```python
from build123d import *

# Parameters (mm, degrees)
F0_R      = 3
F0_R_2    = 13
F1_DEPTH  = 2
F2_R      = 14
F2_R_2    = 12.75
F3_DEPTH  = 2.5
F4_R      = 14
F5_DEPTH  = 2
F7_DEPTH  = 2.5
F9_DEPTH  = 2
F11_DEPTH = 4.5
F12_R     = 24.5
F13_DEPTH = 1


with BuildPart() as f1:
    # F0 (on Top) → F1 (new body)
    with BuildSketch(Plane.XY):
        with BuildLine():
            ThreePointArc((-15, 21.236761), (-26, 0), (-15, -21.236761))
            ThreePointArc((-15, -21.236761), (0, -26), (15, -21.236761))
            ThreePointArc((15, -21.236761), (26, 0), (15, 21.236761))
            ThreePointArc((15, 21.236761), (0, 26), (-15, 21.236761))
        make_face()
        with Locations((0, -19)):
            Circle(F0_R, mode=Mode.SUBTRACT)
        Circle(F0_R_2, mode=Mode.SUBTRACT)
        with Locations((0, 19)):
            Circle(F0_R, mode=Mode.SUBTRACT)
    extrude(amount=F1_DEPTH)

    # F2 (on face) → F3 (join)
    with BuildSketch(Plane.XY.offset(2)):
        Circle(F2_R)
        Circle(F2_R_2, mode=Mode.SUBTRACT)
    extrude(amount=F3_DEPTH)

    # F4 (on face) → F5 (join)
    with BuildSketch(Plane.XY.offset(4.5)):
        Circle(F4_R)
    extrude(amount=F5_DEPTH)

    # F6 (on face) → F7 (join)
    with BuildSketch(Plane.XY.offset(2)):
        with BuildLine():
            Line((23.558438, -11), (19.627786, -11))
            ThreePointArc((19.627786, -11), (22.365353, 2.457846), (16.77051, 15))
            Line((16.77051, 15), (13.228757, 15))
            ThreePointArc((13.228757, 15), (20, 0), (13.228757, -15))
            Line((13.228757, -15), (16.77051, -15))
            Line((16.77051, -15), (21.236761, -15))
            ThreePointArc((21.236761, -15), (22.486717, -13.051726), (23.558438, -11))
        make_face()
        with BuildLine():
            Line((-13.228757, 15), (-16.77051, 15))
            Line((-16.77051, 15), (-21.236761, 15))
            ThreePointArc((-21.236761, 15), (-22.486717, 13.051726), (-23.558438, 11))
            Line((-23.558438, 11), (-19.627786, 11))
            ThreePointArc((-19.627786, 11), (-22.365353, -2.457846), (-16.77051, -15))
            Line((-16.77051, -15), (-13.228757, -15))
            ThreePointArc((-13.228757, -15), (-20, 0), (-13.228757, 15))
        make_face()
    extrude(amount=F7_DEPTH)

    # F8 (on face) → F9 (join)
    with BuildSketch(Plane.XY.offset(4.5)):
        with BuildLine():
            Line((-13.228757, 15), (-21.236761, 15))
            ThreePointArc((-21.236761, 15), (-26, 0), (-21.236761, -15))
            Line((-21.236761, -15), (-13.228757, -15))
            ThreePointArc((-13.228757, -15), (-20, 0), (-13.228757, 15))
        make_face()
        with BuildLine():
            ThreePointArc((21.236761, -15), (26, 0), (21.236761, 15))
            Line((21.236761, 15), (13.228757, 15))
            ThreePointArc((13.228757, 15), (20, 0), (13.228757, -15))
            Line((13.228757, -15), (21.236761, -15))
        make_face()
    extrude(amount=F9_DEPTH)

    # F10 (on face) → F11 (join)
    with BuildSketch(Plane.XY.offset(2)):
        with BuildLine():
            ThreePointArc((-9.177223, 13.106433), (-7.387978, 14.192173), (-5.472322, 15.035082))
            Line((-5.472322, 15.035082), (-7.695453, 21.143084))
            ThreePointArc((-7.695453, 21.143084), (-10.389344, 19.957744), (-12.90547, 18.430921))
            Line((-12.90547, 18.430921), (-9.177223, 13.106433))
        make_face()
        with BuildLine():
            Line((7.695453, 21.143084), (5.472322, 15.035082))
            ThreePointArc((5.472322, 15.035082), (7.387978, 14.192173), (9.177223, 13.106433))
            Line((9.177223, 13.106433), (12.90547, 18.430921))
            ThreePointArc((12.90547, 18.430921), (10.389344, 19.957744), (7.695453, 21.143084))
        make_face()
        with BuildLine():
            Line((-7.695453, -21.143084), (-5.472322, -15.035082))
            ThreePointArc((-5.472322, -15.035082), (-7.387978, -14.192173), (-9.177223, -13.106433))
            Line((-9.177223, -13.106433), (-12.90547, -18.430921))
            ThreePointArc((-12.90547, -18.430921), (-10.389344, -19.957744), (-7.695453, -21.143084))
        make_face()
        with BuildLine():
            ThreePointArc((9.177223, -13.106433), (7.387978, -14.192173), (5.472322, -15.035082))
            Line((5.472322, -15.035082), (7.695453, -21.143084))
            ThreePointArc((7.695453, -21.143084), (10.389344, -19.957744), (12.90547, -18.430921))
            Line((12.90547, -18.430921), (9.177223, -13.106433))
        make_face()
    extrude(amount=F11_DEPTH)

    # F12 (on face) → F13 (cut)
    with BuildSketch(Plane.XY.offset(6.5)):
        Circle(F12_R)
    extrude(amount=-F13_DEPTH, mode=Mode.SUBTRACT)


solid = f1.part
```
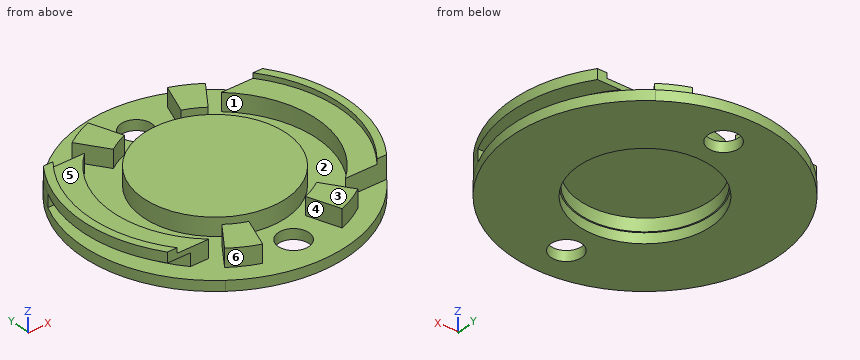
The model under review builds one solid part; all positions refer to its coordinate system, in mm. Face numbers are marked on the shaded views. A direction names the side the tool comes from. Round coordinates to 2 decimals unless told otherwise and drop trailing zeros. Loops run counter-clockwise (first coordinate to the right, second up) from the corner with the lowest first, then second, coordinate; pieces in that order, holes last. Notation, with made-up numbers: (19.25, 3.5) -> (23.25, 3.5) arc R20 ccw to (23.25, 8.5) -> close; hole circle Ø6 at (-21, 14). An arc over 180 degrees is marked (long way). Answer as a JSON object with one key per item and string values. Group by question number.
1) Mouldability with a two-part tool opening along Z and no side actions: class the marked faces 1, 2 and 3 as released by +Z, released by -Z, zero draft, split by the parting line, or undercut.
2) For line 1 (Y direction, x = 0, z = 0.6); line 2 (X direction, y = -0.5, z = 3); line 3 (Y direction, x = -11, z = 2.75), list the stretches that pass through material, from the lowest coordinate up. Write a range as [from, to].
3) For pin 1 Ø2 at (x, y) = (8, 16.5) entering from +Z; pin 2 Ø1 at (x, z) = (-5, 1) entering from +Y; pin 3 Ø13 at (x, y) = (2, 0) entering from -Z; pin 4 Ø10 at (x, y) = (-23, 0) entering from -Z, all flat-tipped, find the tip position at first contact; note any pin that passes through.
4) We need section C-C on x = 11.5. Write out the cut boundary in (y, z), then the cut area to 3 significant figures.
5) For the marked faces 4, 5 and 6, list the 3-axis set-ups (+Z, -Z, +X, -X, +Y, -Y) from which the entire face can be reached by the end or side of a thin tool; tool diameter is ignored.
6) We need section D-D on y = 17. Write out the cut boundary in (x, z), then the cut area to 3 significant figures.
7) We need section A-A on x = 0. Write out the cut boundary in (y, z), then the cut area to 4 significant figures.
Result set:
{
 "1": {"face 1": "zero draft", "face 2": "undercut", "face 3": "released by +Z"},
 "2": {"line 1": "[-26, -22], [-16, -13], [13, 16], [22, 26]", "line 2": "[-22.49, -19.99], [-13.99, -12.74], [12.74, 13.99], [19.99, 22.49]", "line 3": "[-19.63, -15.71], [-8.66, -6.45], [6.45, 8.66], [15.71, 19.63]"},
 "3": {"pin 1": "z = 5.5", "pin 2": "y = 25.61", "pin 3": "z = 4.5", "pin 4": "z = 0"},
 "4": {"outline": "(-23.32, 0) -> (-6.06, 0) -> (-6.06, 2) -> (-5.51, 2) -> (-5.51, 4.5) -> (5.51, 4.5) -> (5.51, 2) -> (6.06, 2) -> (6.06, 0) -> (23.32, 0) -> (23.32, 2) -> (19.34, 2) -> (19.34, 5.5) -> (16.42, 5.5) -> (16.42, 2) -> (7.98, 2) -> (7.98, 5.5) -> (-7.98, 5.5) -> (-7.98, 2) -> (-16.42, 2) -> (-16.42, 5.5) -> (-19.34, 5.5) -> (-19.34, 2) -> (-23.32, 2) -> close", "area": "118 mm²"},
 "5": {"face 4": "+Z, -Y", "face 5": "+Z", "face 6": "+Z, -X, -Y"},
 "6": {"outline": "(-19.67, 0) -> (-2.24, 0) -> (-2.24, 2) -> (-6.19, 2) -> (-6.19, 5.5) -> (-11.9, 5.5) -> (-11.9, 2) -> (-19.67, 2) -> close; (2.24, 0) -> (19.67, 0) -> (19.67, 2) -> (11.9, 2) -> (11.9, 5.5) -> (6.19, 5.5) -> (6.19, 2) -> (2.24, 2) -> close", "area": "110 mm²"},
 "7": {"outline": "(-26, 0) -> (-22, 0) -> (-22, 2) -> (-26, 2) -> close; (-16, 0) -> (-13, 0) -> (-13, 2) -> (-12.75, 2) -> (-12.75, 4.5) -> (12.75, 4.5) -> (12.75, 2) -> (13, 2) -> (13, 0) -> (16, 0) -> (16, 2) -> (14, 2) -> (14, 5.5) -> (-14, 5.5) -> (-14, 2) -> (-16, 2) -> close; (22, 0) -> (26, 0) -> (26, 2) -> (22, 2) -> close", "area": "62.25 mm²"}
}
